The model under review builds one solid part; all positions refer to its coordinate system, in mm. A direction names the side the tool comes from. Round coordinates to 2 decimals unless told otherwise and drop trailing zeros. Order: outer loops, then holes, each group sorted by start corner. A loop starts at its lowest first (then second) coordinate and runs counter-clockwise, first axis right, second up.
1) To check wall thickness, follow L1, parallel to Y at x = -20, z = -7; L2, parallel to X at y = -3, z = 8.5; L3, parallel to X at y = -9.55, z = 1. State the ranges of each line that lie inside material, in increasing order.
2) Consider section B-B (y = -15). Give the boundary of the cut face in (x, z), then the cut area to 3 significant figures.
3) Clearance check with flat-ended pins moving along their axes: P1, Ø2.5, axis at x = 19.5, y = -4, coming from the -Z side; P2, Ø4.5, axis at x = 4, z = 1.5, coming from the -Y side; P3, Ø2, axis at x = -19.5, y = -3.5, coming from the +Z side. State where each tip first meets the part, or that it passes through.
4) Mouldability with a two-part tool opening along Z and no side actions: class faces 4 (the face through (21.65, -4.09, 7.06)), 5 (the face through (4, -4, 3)), 6 (the face through (1.915, -9.042, 2.453)) as pulls with the +Z half, pulls with the -Z half, needs draft (parallel to the pull), parting line crosses it, or undercut.
5) Machinability: for faces 1 (the face through (-22.65, -9.04, 1.09)), 2 (the face through (-18.5, 4, -7)), 3 (the face through (-20, -4, 3)), which of the approach directions +Z, -Z, +X, -X, +Y, -Y give a long, thin tool a straight path to every point of the face, cutting with its end or side? Answer none if there is none.
from build123d import *

# Parameters (mm, degrees)
SKETCH005_W     = 49
SKETCH005_H     = 22
PAD001_DEPTH    = 12
SKETCH006_R     = 2.15
POCKET004_DEPTH = 8
SKETCH007_R     = 2.15
POCKET005_DEPTH = 6
PAD002_DEPTH    = 14
SKETCH009_R     = 2.15
POCKET006_DEPTH = 6
SKETCH010_W     = 3
SKETCH010_H     = 22
PAD003_DEPTH    = 14
POCKET007_DEPTH = 49.001
SKETCH012_R     = 10
PAD004_DEPTH    = 49
SKETCH013_R     = 10
PAD005_DEPTH    = 46
SKETCH014_R     = 7.7
POCKET008_DEPTH = 46.001
SKETCH015_R     = 7.7
POCKET009_DEPTH = 49.001


with BuildPart() as part:
    # Sketch005 → Pad001 (new body)
    with BuildSketch(Plane.XZ):
        Rectangle(SKETCH005_W, SKETCH005_H)
    extrude(amount=PAD001_DEPTH)

    # Sketch006 (on Face1 of Pad001) → Pocket004 (cut)
    with BuildSketch(Plane(origin=(0, 0, 11), x_dir=(-1, 0, 0), z_dir=(0, 0, 1))):
        with Locations((20.5, 4)):
            Circle(SKETCH006_R)
        with Locations((-19.5, 4)):
            Circle(SKETCH006_R)
        with Locations((-3.5, 4)):
            Circle(SKETCH006_R)
    extrude(amount=-POCKET004_DEPTH, mode=Mode.SUBTRACT)

    # Sketch007 (on Face4 of Pocket004) → Pocket005 (cut)
    with BuildSketch(Plane.XZ.offset(12)):
        with Locations((-20.5, 1)):
            Circle(SKETCH007_R)
        with Locations((3.5, 1)):
            Circle(SKETCH007_R)
    extrude(amount=-POCKET005_DEPTH, mode=Mode.SUBTRACT)

    # Sketch008 (on Face8 of Pocket005) → Pad002 (join)
    with BuildSketch(Plane(origin=(0, 0, -11), x_dir=(1, 0, 0), z_dir=(0, 0, -1))):
        Polygon((-24.5, 0), (-24.5, -9.75), (4.5, -9.75), (4.5, -20), (24.5, -20), (24.5, 0), align=None)
    extrude(amount=-PAD002_DEPTH)

    # Sketch009 (on Face10 of Pad002) → Pocket006 (cut)
    with BuildSketch(Plane(origin=(-24.5, 0, 0), x_dir=(0, 0, -1), z_dir=(-1, 0, 0))):
        with Locations((7, -4.25)):
            Circle(SKETCH009_R)
    extrude(amount=-POCKET006_DEPTH, mode=Mode.SUBTRACT)

    # Sketch010 (on Face4 of Pocket006) → Pad003 (join)
    with BuildSketch(Plane.XZ.offset(12)):
        with Locations((23, 0)):
            Rectangle(SKETCH010_W, SKETCH010_H)
    extrude(amount=PAD003_DEPTH)

    # Sketch011 (on Face16 of Pad003) → Pocket007 (cut, through all)
    with BuildSketch(Plane(origin=(24.5, 0, 0), x_dir=(0, 0, 1), z_dir=(1, 0, 0))):
        with BuildLine():
            ThreePointArc((6.984358, 20.901636), (8.634358, 22.551636), (6.984358, 24.201636))
            Line((6.984358, 24.201636), (-0.015642, 24.201636))
            ThreePointArc((-0.015642, 24.201636), (-1.665642, 22.551636), (-0.015642, 20.901636))
            Line((6.984358, 20.901636), (-0.015642, 20.901636))
        make_face()
        with BuildLine():
            ThreePointArc((6.953982, 13.401636), (8.603982, 15.051636), (6.953982, 16.701636))
            Line((6.953982, 16.701636), (-0.046018, 16.701636))
            ThreePointArc((-0.046018, 16.701636), (-1.696018, 15.051636), (-0.046018, 13.401636))
            Line((6.953982, 13.401636), (-0.046018, 13.401636))
        make_face()
    extrude(amount=-POCKET007_DEPTH, mode=Mode.SUBTRACT)

    # Sketch012 (on Face18 of Pocket007) → Pad004 (join)
    with BuildSketch(Plane(origin=(24.5, 0, 0), x_dir=(0, 0, 1), z_dir=(1, 0, 0))):
        with Locations((5, -10)):
            Circle(SKETCH012_R)
    extrude(amount=-PAD004_DEPTH)

    # Sketch013 (on Face40 of Pad004) → Pad005 (join)
    with BuildSketch(Plane(origin=(0, 20, 0), x_dir=(1, 0, 0), z_dir=(0, 1, 0))):
        with Locations((14.5, 13.055578)):
            Circle(SKETCH013_R)
    extrude(amount=-PAD005_DEPTH)

    # Sketch014 (on Face29 of Pad005) → Pocket008 (cut, through all)
    with BuildSketch(Plane(origin=(0, 20, 0), x_dir=(1, 0, 0), z_dir=(0, 1, 0))):
        with Locations((14.5, 13.055578)):
            Circle(SKETCH014_R)
    extrude(amount=-POCKET008_DEPTH, mode=Mode.SUBTRACT)

    # Sketch015 (on Face55 of Pocket008) → Pocket009 (cut, through all)
    with BuildSketch(Plane(origin=(24.5, 0, 0), x_dir=(0, 0, 1), z_dir=(1, 0, 0))):
        with Locations((5, -10)):
            Circle(SKETCH015_R)
    extrude(amount=-POCKET009_DEPTH, mode=Mode.SUBTRACT)


solid = part.part
Answer below:
1. L1: y = -12 to 2.1, 6.4 to 9.75
1. L2: x = -24.5 to -22.4, -18.6 to 1.6, 5.4 to 17.6, 21.4 to 24.5
1. L3: x = -24.5 to -22.65, -18.35 to 1.35, 5.65 to 24.5
2. outline: (21.5, -5.91) arc R10 ccw (long way) to (24.29, -11) - (24.5, -11) - (24.5, -1.7) - (21.5, -1.7) - close; (21.5, 8.6) - (24.5, 8.6) - (24.5, 11) - (21.5, 11) - close; hole circle Ø15.4 at (14.5, -13.06)
2. area: 154 mm2
3. P1: stops at z = -22.33
3. P2: stops at y = -12
3. P3: stops at z = 3
4. face 4: needs draft
4. face 5: pulls with the +Z half
4. face 6: undercut
5. face 1: -Y
5. face 2: -X
5. face 3: +Z
